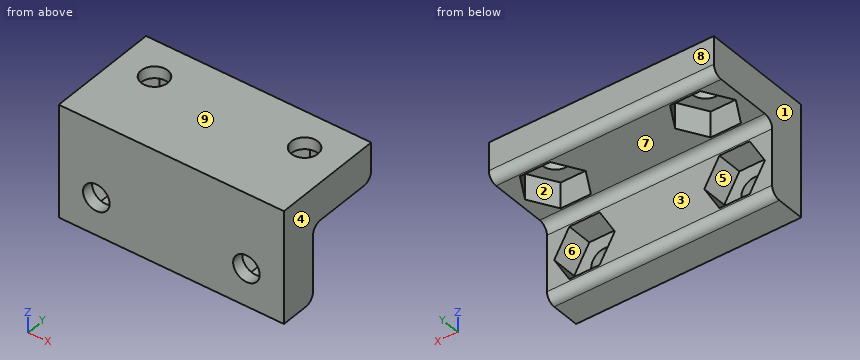
```python
from build123d import *

# Parameters (mm, degrees)
BOSS_EXTRUDE1_DEPTH = 19.05
SKETCH2_R           = 2.2479
CUT_EXTRUDE1_DEPTH  = 4.365625
SKETCH2_2_R         = 2.2479
CUT_EXTRUDE2_DEPTH  = 28.679008291
FILLET1_R           = 1.5875
FILLET2_R           = 1.5875


with BuildPart() as part:
    # Sketch1 → Boss-Extrude1 (new, symmetric)
    with BuildSketch(Plane(origin=(0, 0, 0), x_dir=(0, 0, -1), z_dir=(1, 0, 0))):
        Polygon((0, 0), (6.35, 6.35), (19.05, 6.35), (19.05, 0), align=None)
    extrude(amount=BOSS_EXTRUDE1_DEPTH, both=True)

    # Sketch2 → Cut-Extrude1 (cut)
    # profile 1 of 2: a face of its own
    with BuildSketch(Plane(origin=(0, 6.35, 0), x_dir=(1, 0, 0), z_dir=(0, 1, 0))):
        Polygon((-17.828977719, 12.7), (-15.264488859, 8.258175), (-10.135511141, 8.258175), (-7.571022281, 12.7), (-10.135511141, 17.141825), (-15.264488859, 17.141825), align=None)
        with Locations(Location((-12.7, 12.7, 0), (0, 0, 270))):
            Circle(SKETCH2_R, mode=Mode.SUBTRACT)
    # profile 2 of 2: a face of its own
    with BuildSketch(Plane(origin=(0, 6.35, 0), x_dir=(1, 0, 0), z_dir=(0, 1, 0))):
        Polygon((15.264488859, 17.141825), (17.828977719, 12.7), (15.264488859, 8.258175), (10.135511141, 8.258175), (7.571022281, 12.7), (10.135511141, 17.141825), align=None)
        with Locations(Location((12.7, 12.7, 0), (0, 0, 270))):
            Circle(SKETCH2_R, mode=Mode.SUBTRACT)
    extrude(amount=-CUT_EXTRUDE1_DEPTH, mode=Mode.SUBTRACT)

    # Sketch2_2 → Cut-Extrude2 (cut, through all)
    with BuildSketch(Plane(origin=(0, 6.35, 0), x_dir=(1, 0, 0), z_dir=(0, 1, 0))):
        with Locations(Location((-12.7, 12.7, 0), (0, 0, 270))):
            Circle(SKETCH2_2_R)
        with Locations(Location((12.7, 12.7, 0), (0, 0, 270))):
            Circle(SKETCH2_2_R)
    extrude(amount=-CUT_EXTRUDE2_DEPTH, mode=Mode.SUBTRACT)

    # Mirror1: part across plane


with BuildPart() as part_1:
    add(part.part)
    add(part.part.mirror(Plane(origin=(19.05, 0, 0), x_dir=(0, -0.707106781186549, 0.707106781186546), z_dir=(0, -0.7071067811865462, -0.7071067811865489))))

    # Fillet1
    fillet1_edges = [part_1.edges().sort_by_distance(p)[0] for p in [
        (0, 6.35, -6.35),
    ]]
    fillet(fillet1_edges, radius=FILLET1_R)

    # Fillet2
    fillet2_edges = [part_1.edges().sort_by_distance(p)[0] for p in [
        (0, 19.05, -6.35),
        (0, 6.35, -19.05),
    ]]
    fillet(fillet2_edges, radius=FILLET2_R)


solid = part_1.part
```
Input: part model. Units: mm. Frame: model coordinates. Face numbers are marked on the shaded views. A direction names the side the tool comes from. Give positions to 0.01 mm unless a question says otherwise; leave off trailing zeros. Order: outer loops, then holes, each group sorted by start corner. A loop starts at its lowest first (then second) coordinate and runs counter-clockwise, first axis right, second up. Notation, with made-up numbers: (29.25, -1.5) -> (51.25, -1.5) arc R15 ccw to (51.25, 7.5) -> close; hole circle Ø4 at (40, 19.5). An arc over 180 degrees is marked (long way). Write each question's results on one line, items separated by ' | '. Start each with the question number.
Item 1: Cut plane A-A on x = 12.7. Give the number of separate pieces and of enclosed holes in the cut face, then the cut area to 3 significant figures.
Item 2: Contact query for flat-ended pins moving along their axis: P1, Ø7, axis at x = -10.5, y = 11, coming from the -Z side; P2, Ø7, axis at x = -12.7, y = 12.7, coming from the +Z side; P3, Ø2.5, axis at x = -13, z = -13, coming from the +Y side; P4, Ø6, axis at x = -12.7, z = -12.7, coming from the +Y side. Output: stop coordinate, or through.
Item 3: Line query: line 1 (X direction, y = 0.5, z = -12.7); line 2 (X direction, y = 6, z = -14.5); line 3 (Y direction, x = -13, z = -10). Output: solid intervals per line, ascending.
Item 4: Set-up query: the marked faces 1, 2, 3, 4 and 5. Return all of +Z, -Z, +X, -X, +Y, -Y with unobstructed straight access to the full face (end or side cutting, diameter ignored); none if empty.
Item 5: Cut plane D-D on z = -5.5. Return the cut outline in (x, y).
Item 6: Mould query, pull axis Z, two halves, no side actions, for the marked faces 6, 7, 8 and 9. Classes: pulls with the +Z half, pulls with the -Z half, needs draft (parallel to the pull), parting line crosses it, or undercut.
Item 7: Cut plane B-B on y = 3.25. Return the cut outline in (x, z), then the cut area to 3 significant figures.
Established:
1) separate pieces: 3 | enclosed holes: 0 | area: 106 mm^2
2) P1: z = -6.41 | P2: z = 0 | P3: through | P4: y = 1.98
3) line 1: -19.05 to -14.95, -10.45 to 10.45, 14.95 to 19.05 | line 2: -19.05 to -16.79, -8.61 to 8.61, 16.79 to 19.05 | line 3: 0 to 1.98
4) face 1: +Z, -Z, -X, +Y, -Y | face 2: -Z | face 3: -Z, +X, -X, +Y | face 4: +Z, -Z, +X, +Y, -Y | face 5: +Y
5) outline: (-19.05, 0) -> (19.05, 0) -> (19.05, 18.87) -> (-19.05, 18.87) -> close; hole (-17.83, 12.7) -> (-15.26, 8.26) -> (-10.14, 8.26) -> (-7.57, 12.7) -> (-10.14, 17.14) -> (-15.26, 17.14) -> close; hole (7.57, 12.7) -> (10.14, 8.26) -> (15.26, 8.26) -> (17.83, 12.7) -> (15.26, 17.14) -> (10.14, 17.14) -> close
6) face 6: undercut | face 7: pulls with the -Z half | face 8: needs draft | face 9: pulls with the +Z half
7) outline: (-19.05, -19.05) -> (19.05, -19.05) -> (19.05, 0) -> (-19.05, 0) -> close; hole (-17.83, -12.7) -> (-15.26, -17.14) -> (-10.14, -17.14) -> (-7.57, -12.7) -> (-10.14, -8.26) -> (-15.26, -8.26) -> close; hole (7.57, -12.7) -> (10.14, -17.14) -> (15.26, -17.14) -> (17.83, -12.7) -> (15.26, -8.26) -> (10.14, -8.26) -> close | area: 589 mm^2
